Geometry check sheet. Reference: the model listing, model coordinates, mm. Face numbers are marked on the shaded views. Give positions to 0.01 mm unless a question says otherwise; leave off trailing zeros. Order: outer loops, then holes, each group sorted by start corner. A loop starts at its lowest first (then second) coordinate and runs counter-clockwise, first axis right, second up. Notation, with made-up numbers: M 33,20.5 L 91,20.5 A28 ccw 91,51.5 Z; hole C 67,-28.5 d7. An arc over 180 degrees is marked long. Answer as CSV lines item,"result".
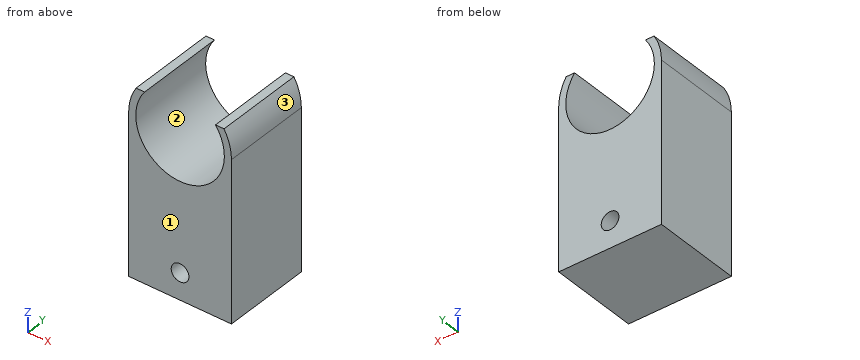
from build123d import *

# Parameters (mm, degrees)
F0_R     = 2.5
F1_DEPTH = 25


with BuildPart() as f1:
    # F0 (on Front) → F1 (new body)
    with BuildSketch(Plane.XZ):
        with BuildLine():
            ThreePointArc((10, 7.5), (0, -12.5), (-10, 7.5))
            Line((-10, 7.5), (-12.409674, 7.5))
            ThreePointArc((-12.409674, 7.5), (-13.967646, 3.892925), (-14.5, 0))
            Line((-14.5, 0), (-14.5, -45))
            Line((-14.5, -45), (14.5, -45))
            Line((14.5, -45), (14.5, 0))
            ThreePointArc((14.5, 0), (13.967646, 3.892925), (12.409674, 7.5))
            Line((12.409674, 7.5), (10, 7.5))
        make_face()
        with Locations((0, -37.5)):
            Circle(F0_R, mode=Mode.SUBTRACT)
    extrude(amount=F1_DEPTH)


solid = f1.part
(1) Material ranges on line 1 (X direction, y = -17, z = 0); line 2 (Z direction, x = 11, y = -11.25); line 3 (X direction, y = -16.5, z = -9), recorded low to high.
The answers:
line 1,"x = -14.5 to -12.5, 12.5 to 14.5"
line 2,"z = -45 to -5.94, 5.94 to 7.5"
line 3,"x = -14.5 to -8.67, 8.67 to 14.5"
(2) Section check C-C on z = -37.5. Enter the section's corners in (x, y), then the cut area to 3 significant figures.
The answers:
outline,"M -14.5,-25 L -2.5,-25 L -2.5,0 L -14.5,0 Z; M 2.5,-25 L 14.5,-25 L 14.5,0 L 2.5,0 Z"
area,"600 mm2"
(3) Section check B-B on y = -14. Enter the section's corners in (x, z).
The answers:
outline,"M -14.5,-45 L 14.5,-45 L 14.5,0 A14.5 ccw 12.41,7.5 L 10,7.5 A12.5 cw long -10,7.5 L -12.41,7.5 A14.5 ccw -14.5,0 Z; hole C 0,-37.5 d5"
(4) Draft check along Z on the marked faces 1, 2 and 3. Enter one of: +Z half, -Z half, draft (parallel to the pull), parting line (faces both ways), or undercut.
The answers:
face 1,"draft"
face 2,"undercut"
face 3,"+Z half"
(5) Gauge pin test, flat end, axial feed: P1, Ø1, axis at y = -9.5, z = 0.5, coming from the +X side. Record the tip position at first contact, or that the pin passes through.
The answers:
P1,"stops at x = 14.5"
(6) Section check A-A on x = 0. Enter the section's corners in (y, z).
The answers:
outline,"M -25,-45 L 0,-45 L 0,-40 L -25,-40 Z; M -25,-35 L 0,-35 L 0,-12.5 L -25,-12.5 Z"
